The listing builds one solid part. Answer for the finished solid, in the listing's coordinates (mm). Face numbers are marked on the shaded views. A direction names the side the tool comes from. Round coordinates to 2 decimals unless told otherwise and drop trailing zeros. Loops run counter-clockwise (first coordinate to the right, second up) from the corner with the lowest first, then second, coordinate; pieces in that order, holes last. Notation, with made-up numbers: (-27, -14.75) -> (-8, -14.75) arc R25 ccw to (-8, 4.25) -> close; hole circle Ø1 at (-17.5, 26.5). An arc over 180 degrees is marked (long way). Write each question's results on one line, items separated by ' | '. Start each with the question number.
(1) Straight lines are drawn through the part: probe 1 along Y at (x, z) = (88.25, 0); probe 2 along X at (y, z) = (-17.5, 9.5); probe 3 along X at (y, z) = (41, -21.5). For each, find the intervals that lie inside material, in ascending order.
(2) The part is cut by section A-A (y = -40.9). Determine the outline of the cut face in (x, z).
(3) Flat-ended cylindrical pins translate along their axes: pin 1 (5 mm diameter, centred on x = 85, y = -3.5, fed in from +Z); pin 2 (3 mm diameter, centred on x = 73.5, z = -15, fed in from -Y); pin 3 (5 mm diameter, centred on y = 40.84, z = 45.82, fed in from +X); pin 4 (3 mm diameter, centred on y = 17, z = -15, fed in from +X). Find the tip coordinate at first contact, or state that the pin passes through.
(4) The part is cut by section D-D (y = 0). Determine the outline of the cut face in (x, z), plus the area to 3 significant figures.
(5) The part is cut by section C-C (x = 37). Determine the outline of the cut face in (y, z), plus the area to 3 significant figures.
(6) The part is cut by section B-B (x = 78). Determine the outline of the cut face in (y, z), plus the area to 3 significant figures.
(7) Determine the mould class of the marked faces 3, 4, 5 and 6 for opening direction Z: released by +Z, released by -Z, zero draft, split by the parting line, or undercut.
(8) For the marked faces 1 and 2, determine the directions among +Z, -Z, +X, -X, +Y, -Y from which every point of the face is accessible in a straight line to the end or side of a thin tool.
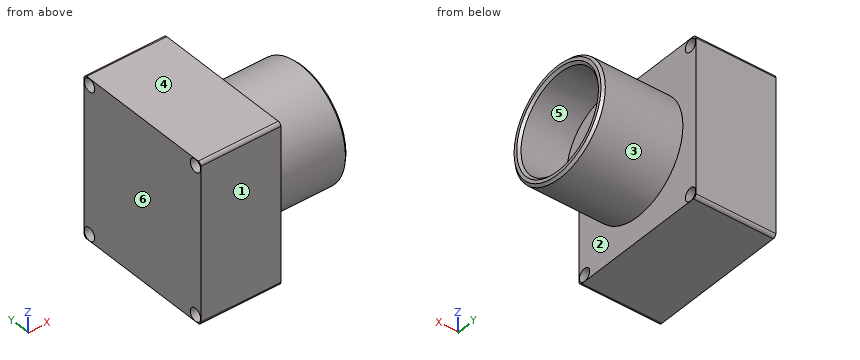
Autodesk Inventor part; units mm, degrees
ref_plane "YZ Plane" through (0, 0, 0) normal (1, 0, 0) x (0, 1, 0)
ref_plane "XZ Plane" through (0, 0, 0) normal (0, 1, 0) x (-1, 0, 0)
ref_plane "XY Plane" through (0, 0, 0) normal (0, 0, 1) x (1, 0, 0)
sketch "Boceto1" plane through (0, 0, 0) normal (1, 0, 0) x (0, 1, 0)
  line L0 (-45, -50) -> (45, -50)
  line L1 (45, -50) -> (45, 50)
  line L2 (45, 50) -> (-45, 50)
  line L3 (-45, 50) -> (-45, -50)
  line L4 (-45, -50) -> (45, 50) construction
  line L5 (45, -50) -> (-45, 50) construction
  point P0 (0, 0)
  dimension "d0" = 90
  dimension "d1" = 100
extrude "Extrusión1" add sketch "Boceto1" along normal blind 50
sketch "Boceto2" plane through (50, 0, 0) normal (1, 0, 0) x (0, 0, -1)
  circle A0 centre (0, 0) radius 35
  dimension "d4" = 70
extrude "Extrusión2" add sketch "Boceto2" along normal blind 50
sketch "Boceto3" plane through (100, 0, 0) normal (1, 0, 0) x (0, 0, -1)
  circle A0 centre (0, 0) radius 30
  dimension "d7" = 60
extrude "Extrusión3" cut sketch "Boceto3" against normal blind 30
chamfer "Chaflán1" distance 1.5 angle 45 2 edges at (100, 0, 35) (100, 0, 30)
sketch "Boceto4" plane through (50, 0, 0) normal (1, 0, 0) x (0, 0, -1)
  point P0 (0, 0)
fillet "Empalme1" radius 2 4 edges at (25, 45, 50) (25, -45, 50) (25, 45, -50) (25, -45, -50)
sketch "Boceto5" plane through (50, 0, 0) normal (1, 0, 0) x (0, 0, -1)
  point P0 (0, 0)
  point P1 (-45.8189, 40.8434)
hole "Agujero1" at (50, 40.8434, 45.8189) direction (-1, 0, 0) diameter 8 end through all
sketch "Boceto6" plane through (50, 0, 0) normal (1, 0, 0) x (0, 0, -1)
  line L0 (48, 45) -> (-48, 45)
  point P0 (0, 0)
  point P1 (45.9279, 40.9)
  dimension "d21" = 4.1
hole "Agujero2" at (50, 40.9, -45.9279) direction (-1, 0, 0) diameter 8 end through all
sketch "Boceto7" plane through (50, 0, 0) normal (1, 0, 0) x (0, 0, -1)
  line L0 (-48, -45) -> (48, -45)
  point P0 (0, 0)
  point P1 (-45.9235, -40.9)
  dimension "d29" = 4.1
hole "Agujero3" at (50, -40.9, 45.9235) direction (-1, 0, 0) diameter 8 end through all
sketch "Boceto8" plane through (50, 0, 0) normal (1, 0, 0) x (0, 0, -1)
  line L0 (-48, -45) -> (48, -45)
  point P0 (0, 0)
  point P1 (45.9358, -40.9)
  dimension "d37" = 4.1
hole "Agujero4" at (50, -40.9, -45.9358) direction (-1, 0, 0) diameter 8 end through all
properties part number "TAREA 1 LAB DINAMICA 1168717"
Checked values:
1) probe 1: y = -35 to -30, 30 to 35 | probe 2: x = 0 to 70 | probe 3: x = 0 to 50
2) outline: (0, -50) -> (50, -50) -> (50, -49.94) -> (0, -49.94) -> close; (0, -41.94) -> (50, -41.94) -> (50, 41.92) -> (0, 41.92) -> close; (0, 49.92) -> (50, 49.92) -> (50, 50) -> (0, 50) -> close
3) pin 1: stops at z = 34.99 | pin 2: stops at y = -32.29 | pin 3: passes through | pin 4: stops at x = 70
4) outline: (0, -50) -> (50, -50) -> (50, -35) -> (98.5, -35) -> (100, -33.5) -> (100, -31.5) -> (98.5, -30) -> (70, -30) -> (70, 30) -> (98.5, 30) -> (100, 31.5) -> (100, 33.5) -> (98.5, 35) -> (50, 35) -> (50, 50) -> (0, 50) -> close | area: 6,700 mm2
5) outline: (-45, -48) arc R2 ccw to (-43, -50) -> (43, -50) arc R2 ccw to (45, -48) -> (45, 48) arc R2 ccw to (43, 50) -> (-43, 50) arc R2 ccw to (-45, 48) -> close; hole circle Ø8 at (-40.9, -45.94); hole circle Ø8 at (-40.9, 45.92); hole circle Ø8 at (40.84, 45.82); hole circle Ø8 at (40.9, -45.93) | area: 8,800 mm2
6) outline: circle Ø70 at (0, 0); hole circle Ø60 at (0, 0) | area: 1,020 mm2
7) face 3: split by the parting line | face 4: released by +Z | face 5: undercut | face 6: zero draft
8) face 1: +Z, -Z, +X, -X, -Y | face 2: +X
